Autodesk Inventor part; units mm, degrees
ref_plane "Work Plane1" through (30, 0, 2.5) normal (-1, 0, 0) x (0, 0, 1)
ref_plane "YZ Plane" through (0, 0, 0) normal (1, 0, 0) x (0, 1, 0)
ref_plane "XZ Plane" through (0, 0, 0) normal (0, 1, 0) x (-1, 0, 0)
sketch "Sketch1" plane through (0, 0, 0) normal (0, 0, 1) x (1, 0, 0)
  line L0 (0, 0) -> (60, 0)
  line L1 (60, 0) -> (60, 10)
  line L2 (60, 10) -> (0, 10)
  line L3 (0, 10) -> (0, 0)
  line L4 (30, 10) -> (30, 0) construction
  dimension "d0" = 60
  dimension "d2" = 10
extrude "Extrusion1" add sketch "Sketch1" along normal mid plane 5
sketch "Sketch2" plane through (0, 0, 2.5) normal (0, 0, 1) x (1, 0, 0)
  circle A0 centre (5, 5) radius 3.45
  line L0 (60, 10) -> (0, 10)
  line L1 (60, 0) -> (60, 10)
  line L2 (60, 10) -> (0, 10)
  line L3 (0, 10) -> (0, 0)
  line L4 (0, 0) -> (60, 0)
  line L5 (7.2091, 7.65) -> (7.2091, 2.35) construction
  arc A1 (19.1591, 3.003) -> (19.1591, 6.997) centre (19.05, 5) ccw
  line L6 (7.2091, 7.65) -> (19.1591, 6.997)
  line L7 (5, 5) -> (19.05, 5) construction
  line L8 (7.2091, 2.35) -> (19.1591, 3.003)
  line L9 (0, 5) -> (5, 5) construction
  line L10 (5, 10) -> (5, 5) construction
  dimension "d8" = 6.9
  dimension "d9" = 5.3
  dimension "d10" = 14.05
  dimension "d11" = 2
extrude "Extrusion2" cut sketch "Sketch2" along normal through all both and the other way through all contours A0
extrude "Extrusion3" cut sketch "Sketch2" against normal blind 1.4 contours A0 L6 A1 L8
ref_plane "Work Plane1" through (30, 0, 2.5) normal (-1, 0, 0) x (0, 0, 1)
mirror "Mirror1" about plane through (30, 0, 2.5) normal (-1, 0, 0) of "Extrusion2", "Extrusion3"
fillet "Fillet1" radius 2 4 edges at (60, 10, 0) (60, 0, 0) (0, 0, 0) (0, 10, 0)
sketch "Sketch3" plane through (0, 0, 2.5) normal (0, 0, 1) x (1, 0, 0)
  line L0 (30, -2) -> (30, 12)
  line L1 (0, 8) -> (0, 2)
  line L2 (23.05, 7) -> (36.95, 7)
  line L3 (36.95, 7) -> (36.95, 3)
  line L4 (36.95, 3) -> (23.05, 3)
  line L5 (23.05, 3) -> (23.05, 7)
  line L6 (23.05, 7) -> (36.95, 3) construction
  line L7 (36.95, 7) -> (23.05, 3) construction
  arc A0 (40.8409, 6.997) -> (40.8409, 3.003) centre (40.95, 5) ccw construction
  line L8 (58, 10) -> (2, 10) construction
  line L9 (30, 7) -> (30, 10) construction
  line L10 (2, 0) -> (58, 0)
  point P0 (0, 0)
  point P1 (30, 5)
  point P2 (38.95, 5)
  point P3 (0, 5)
  dimension "d26" = 2
  dimension "d27" = 3
extrude "Extrusion4" cut sketch "Sketch3" against normal through all
fillet "Fillet2" radius 1 4 edges at (23.05, 7, 0) (23.05, 3, 0) (36.95, 3, 0) (36.95, 7, 0)
properties part number "leg_v0.1"
Could you check a few things on this model? Use its own coordinates, in mm. A direction names the side the tool comes from. Round coordinates to 2 decimals unless told otherwise and drop trailing zeros. Loops run counter-clockwise (first coordinate to the right, second up) from the corner with the lowest first, then second, coordinate; pieces in that order, holes last.
Q1. I want a section at B-B (y = 5). Write out the boundary of the cut face in (x, z).
Q2. I want a section at A-A (x = 31). Write out the boundary of the cut face in (y, z), and give its area (3 significant figures).
Q3. I want a section at D-D (x = 43). Write out the boundary of the cut face in (y, z).
Q4. For P1, Ø1.6, axis at x = 17.5, y = 5, coming from the +Z side, with a flat end and sliding along its axis, tell me the tip position at first contact or that it passes through.
Q5. Please list where these lines run through material, in increasing order: L1, parallel to X at y = 5, z = -1.4; L2, parallel to Y at x = 55, z = -1.45; L3, parallel to Y at x = 28.5, z = -0.1.
Q6. I want a section at C-C (z = -1). Write out the boundary of the cut face in (x, y), and give its area (3 significant figures).
Q7. Thinking about a two-plate mould opening in X: for faces 4 (the flat face through (29.6, 7.3, 2.5)), 5 (the cylindrical face through (36.649, 6.715, -0.035)), 6 (the cylindrical face through (0.57, 0.6, 0.04)), which applies, pulls with the +X half, pulls with the -X half, needs draft (parallel to the pull), parting line crosses it, or undercut?
Q8. On a 3-axis mill with a long thin cutter (end or side, diameter ignored), from which of +Z, -Z, +X, -X, +Y, -Y can I reach the whole of each face in a straight line? I mean faces 1 (the flat face through (36.95, 5, 0)), 2 (the flat face through (14, 5, 1.1)), 3 (the flat face through (30, 0, 0)). Say none if no direction works.
Answer below:
1. outline: (0, -2.5) - (1.55, -2.5) - (1.55, 2.5) - (0, 2.5) - close; (8.45, -2.5) - (23.05, -2.5) - (23.05, 2.5) - (21.05, 2.5) - (21.05, 1.1) - (8.45, 1.1) - close; (36.95, -2.5) - (51.55, -2.5) - (51.55, 1.1) - (38.95, 1.1) - (38.95, 2.5) - (36.95, 2.5) - close; (58.45, -2.5) - (60, -2.5) - (60, 2.5) - (58.45, 2.5) - close
2. outline: (0, -2.5) - (3, -2.5) - (3, 2.5) - (0, 2.5) - close; (7, -2.5) - (10, -2.5) - (10, 2.5) - (7, 2.5) - close
2. area: 30.0 mm2
3. outline: (0, -2.5) - (10, -2.5) - (10, 2.5) - (7.11, 2.5) - (7.11, 1.1) - (2.89, 1.1) - (2.89, 2.5) - (0, 2.5) - close
4. P1: stops at z = 1.1
5. L1: x = 0 to 1.55, 8.45 to 23.05, 36.95 to 51.55, 58.45 to 60
5. L2: y = 0 to 1.55, 8.45 to 10
5. L3: y = 0 to 3, 7 to 10
6. outline: (0, 2) arc R2 ccw to (2, 0) - (58, 0) arc R2 ccw to (60, 2) - (60, 8) arc R2 ccw to (58, 10) - (2, 10) arc R2 ccw to (0, 8) - close; hole circle Ø6.9 at (5, 5); hole (23.05, 4) arc R1 ccw to (24.05, 3) - (35.95, 3) arc R1 ccw to (36.95, 4) - (36.95, 6) arc R1 ccw to (35.95, 7) - (24.05, 7) arc R1 ccw to (23.05, 6) - close; hole circle Ø6.9 at (55, 5)
6. area: 467 mm2
7. face 4: needs draft
7. face 5: undercut
7. face 6: pulls with the -X half
8. face 1: +Z, -Z
8. face 2: +Z
8. face 3: +Z, -Z, +X, -X, -Y
